Design review of the part built by this model. Coordinates are the model's own, in mm. Face numbers are marked on the shaded views. Round coordinates to 2 decimals unless told otherwise and drop trailing zeros. Order: outer loops, then holes, each group sorted by start corner. A loop starts at its lowest first (then second) coordinate and runs counter-clockwise, first axis right, second up. Notation, with made-up numbers: (-10, 87.5) - (47, 87.5) arc R21 ccw to (47, 109.5) - close; hole circle Ø8 at (-1.5, 52.25). An arc over 180 degrees is marked (long way). Write item = value, one per line.
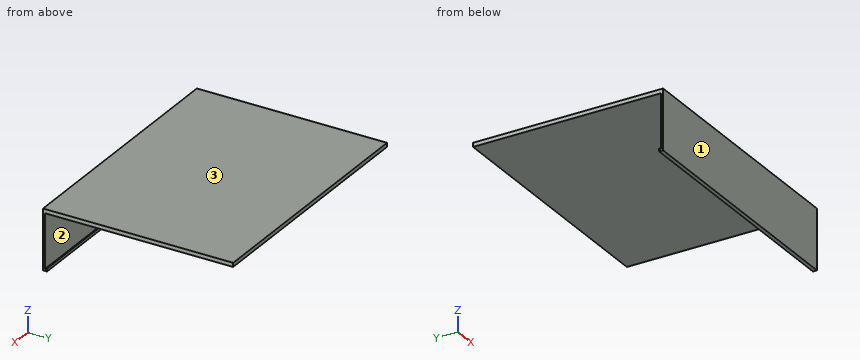
Autodesk Inventor part; units mm, degrees
ref_plane "YZ Plane" through (0, 0, 0) normal (1, 0, 0) x (0, 1, 0)
ref_plane "XZ Plane" through (0, 0, 0) normal (0, 1, 0) x (-1, 0, 0)
ref_plane "XY Plane" through (0, 0, 0) normal (0, 0, 1) x (1, 0, 0)
sketch "草圖1" plane through (0, 0, 0) normal (0, 1, 0) x (-1, 0, 0)
  line L0 (0, 0) -> (-254, 0)
  line L1 (-254, 0) -> (-254, 60)
  line L2 (-254, 60) -> (0, 60)
  line L3 (0, 60) -> (0, 0)
  dimension "d0" = 254
  dimension "d1" = 60
extrude "擠出1" add sketch "草圖1" along normal blind 190
sketch "草圖2" plane through (0, 190, 0) normal (0, 1, 0) x (1, 0, 0)
  line L0 (254, 0) -> (0, 0)
  line L1 (0, 0) -> (254, 0)
  line L2 (254, 0) -> (254, -56)
  line L3 (254, -56) -> (0, -56)
  line L4 (0, -56) -> (0, 0)
  dimension "d4" = 254
  dimension "d5" = 56
extrude "擠出2" cut sketch "草圖2" against normal blind 188
sketch "草圖3" plane through (0, 2, 0) normal (0, 1, 0) x (1, 0, 0)
  line L0 (0, 0) -> (254, 0)
  line L1 (254, 0) -> (254, -2)
  line L2 (254, -2) -> (0, -2)
  line L3 (0, -2) -> (0, 0)
  dimension "d8" = 254
  dimension "d9" = 2
extrude "擠出3" add sketch "草圖3" along normal blind 2
sketch "草圖4" plane through (0, 2, 2) normal (0, 0, 1) x (1, 0, 0)
  line L0 (0, 2) -> (254, 2)
  line L1 (0, 2) -> (254, 2)
  line L2 (254, 2) -> (254, 1.2)
  line L3 (254, 1.2) -> (0, 1.2)
  line L4 (0, 1.2) -> (0, 2)
  point P0 (0, -2)
  dimension "d12" = 254
  dimension "d13" = 0.8
extrude "擠出4" add sketch "草圖4" along normal blind 0.8
properties part number "包包分隔檔板"
Item 1: For line 1 along Z through (x, y) = (165.5, 124); line 2 along Y through (x, z) = (202.5, 7), list the stretches that pass through material, from the lowest coordinate up. Write a range as [from, to].
Data:
line_1 = [56, 60]
line_2 = [0, 2]
Item 2: Insertion check: P1, Ø1, axis at x = 200.5, y = 160, coming from the -Z side; P2, Ø12, axis at x = 134.5, z = 11.5, coming from the +Y side; P3, Ø0.8, axis at x = 153, z = 1, coming from the +Y side. Each pin has a flat end and moves straight along its axis. Give the tip position at first contact, or say it passes through.
Data:
P1 = 56
P2 = 2
P3 = 4
Item 3: Take a section at B-B, the plane z = 28. State the section outline as (x, y) points.
Data:
outline = (0, 0) - (254, 0) - (254, 2) - (0, 2) - close
Item 4: Take a section at A-A, the plane x = 117. State the section outline as (y, z) points.
Data:
outline = (0, 0) - (4, 0) - (4, 2.8) - (3.2, 2.8) - (3.2, 2) - (2, 2) - (2, 56) - (190, 56) - (190, 60) - (0, 60) - close
Item 5: Take a section at C-C, the plane y = 171. State the section outline as (x, z) points, and give its area (3 significant figures).
Data:
outline = (0, 56) - (254, 56) - (254, 60) - (0, 60) - close
area = 1,020 mm2
Item 6: The part is to be moulded in two halves that separate along Z. For the marked faces 1, 2 and 3, say which applies: +Z half, -Z half, draft (parallel to the pull), parting line (faces both ways), or undercut.
Data:
face_1 = draft
face_2 = undercut
face_3 = +Z half
